Source: CAD feature listing. Evaluate the final solid. Frame: model axes, mm. A direction names the side the tool comes from. Coordinates: 2 decimals unless noted, no trailing zeros. Order: outer loops, then holes, each group sorted by start corner. A loop starts at its lowest first (then second) coordinate and runs counter-clockwise, first axis right, second up. Notation, with made-up numbers: (84, 44.25) -> (96, 44.25) arc R22 cw to (96, 64.25) -> close; hole circle Ø3 at (-3.5, 0). An arc over 180 degrees is marked (long way). Write each question's results on one line, items separated by ' | '. Start each with the question number.
from build123d import *

# Parameters (mm, degrees)
F1_DEPTH = 2
F2_R     = 1.5
F3_R     = 0.4


with BuildPart() as f1:
    # F0 (on Top) → F1 (new body)
    with BuildSketch(Plane.XY):
        with BuildLine():
            ThreePointArc((-7.2316509448, 2.5), (-4.1547013841, 2.6433820369), (-2.5733385496, 0))
            ThreePointArc((-2.5733385496, 0), (-4.1547013841, -2.6433820369), (-7.2316509448, -2.5))
            Line((-7.2316509448, -2.5), (-11.7673134743, -2.5))
            ThreePointArc((-11.7673134743, -2.5), (-13.7940116366, -4.6904157598), (-16.6662929599, -5.5))
            Line((-16.6662929599, -5.5), (16.6662929599, -5.5))
            ThreePointArc((16.6662929599, -5.5), (13.7940116366, -4.6904157598), (11.7673134743, -2.5))
            Line((11.7673134743, -2.5), (7.2316509448, -2.5))
            ThreePointArc((7.2316509448, -2.5), (2.5733385496, 0), (7.2316509448, 2.5))
            Line((7.2316509448, 2.5), (11.7673134743, 2.5))
            ThreePointArc((11.7673134743, 2.5), (13.7940116366, 4.6904157598), (16.6662929599, 5.5))
            Line((16.6662929599, 5.5), (-16.6662929599, 5.5))
            ThreePointArc((-16.6662929599, 5.5), (-13.7940116366, 4.6904157598), (-11.7673134743, 2.5))
            Line((-11.7673134743, 2.5), (-7.2316509448, 2.5))
        make_face()
        with BuildLine():
            Line((-15.0079805647, 2.5), (-11.7673134743, 2.5))
            ThreePointArc((-11.7673134743, 2.5), (-13.7940116366, 4.6904157598), (-16.6662929599, 5.5))
            ThreePointArc((-16.6662929599, 5.5), (-19.5385742831, 4.6904157598), (-21.5652724454, 2.5))
            Line((-21.5652724454, 2.5), (-18.324605355, 2.5))
            ThreePointArc((-18.324605355, 2.5), (-16.6662929599, 3), (-15.0079805647, 2.5))
        make_face()
        with BuildLine():
            ThreePointArc((-16.6662929599, -5.5), (-13.7940116366, -4.6904157598), (-11.7673134743, -2.5))
            Line((-11.7673134743, -2.5), (-15.0079805647, -2.5))
            ThreePointArc((-15.0079805647, -2.5), (-16.6662929599, -3), (-18.324605355, -2.5))
            Line((-18.324605355, -2.5), (-21.5652724454, -2.5))
            ThreePointArc((-21.5652724454, -2.5), (-19.5385742831, -4.6904157598), (-16.6662929599, -5.5))
        make_face()
        with BuildLine():
            ThreePointArc((21.5652724454, 2.5), (19.5385742831, 4.6904157598), (16.6662929599, 5.5))
            ThreePointArc((16.6662929599, 5.5), (13.7940116366, 4.6904157598), (11.7673134743, 2.5))
            Line((11.7673134743, 2.5), (15.0079805647, 2.5))
            ThreePointArc((15.0079805647, 2.5), (16.6662929599, 3), (18.324605355, 2.5))
            Line((18.324605355, 2.5), (21.5652724454, 2.5))
        make_face()
        with BuildLine():
            ThreePointArc((11.7673134743, -2.5), (13.7940116366, -4.6904157598), (16.6662929599, -5.5))
            ThreePointArc((16.6662929599, -5.5), (19.5385742831, -4.6904157598), (21.5652724454, -2.5))
            Line((21.5652724454, -2.5), (18.324605355, -2.5))
            ThreePointArc((18.324605355, -2.5), (16.6662929599, -3), (15.0079805647, -2.5))
            Line((15.0079805647, -2.5), (11.7673134743, -2.5))
        make_face()
    extrude(amount=F1_DEPTH)

    # F2
    f2_edges = [f1.edges().sort_by_distance(p)[0] for p in [
        (-15.007981, 2.5, 1),
        (-18.324605, 2.5, 1),
        (-7.231651, 2.5, 1),
        (-18.324605, -2.5, 1),
        (-15.007981, -2.5, 1),
        (-7.231651, -2.5, 1),
        (7.231651, 2.5, 1),
        (18.324605, 2.5, 1),
        (15.007981, 2.5, 1),
        (7.231651, -2.5, 1),
        (15.007981, -2.5, 1),
        (18.324605, -2.5, 1),
    ]]
    fillet(f2_edges, radius=F2_R)

    # F3
    f3_edges = [f1.edges().sort_by_distance(p)[0] for p in [
        (21.565272, 2.5, 1),
        (21.565272, -2.5, 1),
        (-21.565272, 2.5, 1),
        (-21.565272, -2.5, 1),
    ]]
    fillet(f3_edges, radius=F3_R)


solid = f1.part
(1) Draft query along X for faces 1 (the cylindrical face through (19.253, 4.853, 0.986)), 2 (the cylindrical face through (-16.6, -3, 1)), 3 (the flat face through (-11, -2.5, 1)). Return one class per face: released by +X, released by -X, zero draft, split by the parting line, or undercut.
(2) Section C-C on y = -2. Return the cut outline in (x, z).
(3) Section A-A on x = 6. Return the cut outline in (y, z), then the cut area to 3 significant figures.
(4) Section D-D on y = 4. Return the cut outline in (x, z), then the cut area to 3 significant figures.
(5) Section B-B on x = -16. Return the cut outline in (y, z).
(6) Line query: L1, parallel to X at y = -2.75, z = 0.2; L2, parallel to Y at x = 10.5, z = 1.65; L3, parallel to X at y = 0, z = 1.5. Output: solid intervals per line, ascending.
(7) First-contact query: P1, Ø1, axis at x = -20, z = 1.5, coming from the -Y side; P2, Ø0.6, axis at x = -20, z = 1.5, coming from the +Y side. Flat tips, straight axial feed; report the tip coordinate or a pass-through.
(8) Reachability of faces 4 (the flat face through (0, 5.5, 1)), 5 (the flat face through (20, 2.5, 1)), 6 (the flat face through (-20, 2.5, 1)), 7 (the cylindrical face through (16.7, -3, 1)), 8 (the flat face through (0, 0, 0)) from +Z, -Z, +X, -X, +Y, -Y: full face, straight path, thin tool, end or side. Return the list, or none.
Results list:
1) face 1: released by +X | face 2: undercut | face 3: zero draft
2) outline: (-3.34, 0) -> (3.34, 0) -> (3.34, 2) -> (-3.34, 2) -> close
3) outline: (-5.5, 0) -> (-2.97, 0) -> (-2.97, 2) -> (-5.5, 2) -> close; (2.97, 0) -> (5.5, 0) -> (5.5, 2) -> (2.97, 2) -> close | area: 10.1 mm²
4) outline: (-20.44, 0) -> (20.44, 0) -> (20.44, 2) -> (-20.44, 2) -> close | area: 81.8 mm²
5) outline: (-5.5, 0) -> (-2.93, 0) -> (-2.93, 2) -> (-5.5, 2) -> close; (2.93, 0) -> (5.5, 0) -> (5.5, 2) -> (2.93, 2) -> close
6) L1: x = -21.23 to -17.87, -15.47 to -6.77, -4.37 to 4.37, 6.77 to 15.47, 17.87 to 21.23 | L2: y = -5.5 to -2.5, 2.5 to 5.5 | L3: x = -2.57 to 2.57
7) P1: stops at y = -4.71 | P2: stops at y = 4.59
8) face 4: +Z, -Z, +X, -X, +Y | face 5: +Z, -Z, +X | face 6: +Z, -Z, -X | face 7: +Z, -Z | face 8: -Z, +X, -X, +Y, -Y
